CAD build for the part. Positions are in the model's coordinates, mm. Face numbers are marked on the shaded views. Give positions to 0.01 mm unless a question says otherwise; leave off trailing zeros. Order: outer loops, then holes, each group sorted by start corner. A loop starts at its lowest first (then second) coordinate and runs counter-clockwise, first axis right, second up.
Item 1: Two-plate mould, pull along X, no slides. Class the marked faces 1, 2 and 3: released by +X, released by -X, zero draft, split by the parting line, or undercut.
Item 2: Wall check: L1, parallel to Y at x = -1.8, z = 5.5; L2, parallel to Y at x = 1.3, z = -3.8; L3, parallel to Z at x = -0.25, y = 6. Give the ranges that are in metal, low to high.
Item 3: Band-saw the part on B-B on z = 7.75. Give the cut face in (x, y).
Item 4: Band-saw the part on C-C on y = 0. Give the cut face in (x, z), plus the area to 3 significant figures.
Item 5: Flat gauge pins, fed straight in: P1, Ø6.5, axis at x = -2.5, y = 3, coming from the -Z side; P2, Ø6, axis at y = -3, z = 2, coming from the +X side; P3, Ø0.6, axis at y = 0, z = -1.5, coming from the +X side. Where does each tip first touch, or does it go through?
Item 6: Band-saw the part on A-A on z = -3.8. Give the cut face in (x, y), plus the area to 3 significant figures.
```python
from build123d import *

# Parameters (mm, degrees)
ESQUISSE1_R             = 7
BOSS_EXTRU_1_DEPTH      = 12.5
ESQUISSE2_R             = 7
ESQUISSE2_R_2           = 6.4
ENL_V_MAT_EXTRU_1_DEPTH = 10.5
ESQUISSE4_R             = 3.15
ENL_V_MAT_EXTRU_3_DEPTH = 9
ESQUISSE5_R             = 0.8
BOSS_EXTRU_2_DEPTH      = 8.5
ESQUISSE6_W             = 0.5
ESQUISSE6_H             = 2
BOSS_EXTRU_3_DEPTH      = 5
ESQUISSE7_R             = 0.5
ENL_V_MAT_EXTRU_4_DEPTH = 9.587227572
ESQUISSE8_R             = 0.5
ENL_V_MAT_EXTRU_5_DEPTH = 12.087439586
CONG_7_R                = 0.8


with BuildPart() as part:
    # Esquisse1 → Boss.-Extru.1 (new body)
    with BuildSketch(Plane.XY):
        Circle(ESQUISSE1_R)
    extrude(amount=BOSS_EXTRU_1_DEPTH)

    # Esquisse2 → Enlèv. mat.-Extru.1 (cut)
    with BuildSketch(Plane(origin=(0, 0, 0), x_dir=(-1, 0, 0), z_dir=(0, 0, -1))):
        Circle(ESQUISSE2_R)
        Circle(ESQUISSE2_R_2, mode=Mode.SUBTRACT)
    extrude(amount=-ENL_V_MAT_EXTRU_1_DEPTH, mode=Mode.SUBTRACT)

    # Esquisse4 → Enlèv. mat.-Extru.3 (cut)
    with BuildSketch(Plane.XY.offset(12.5)):
        with Locations((-1.8, 0)):
            Circle(ESQUISSE4_R)
    extrude(amount=-ENL_V_MAT_EXTRU_3_DEPTH, mode=Mode.SUBTRACT)

    # Esquisse5 → Boss.-Extru.2 (add)
    with BuildSketch(Plane.XY.offset(3.5)):
        with Locations((-1.8, 0)):
            Circle(ESQUISSE5_R)
    extrude(amount=BOSS_EXTRU_2_DEPTH)

    # Esquisse6 → Boss.-Extru.3 (add)
    with BuildSketch(Plane(origin=(0, 0, 0), x_dir=(-1, 0, 0), z_dir=(0, 0, -1))):
        with Locations((-3.837439586, 0)):
            Rectangle(ESQUISSE6_W, ESQUISSE6_H)
        with Locations((-1.337227572, -3.389935619)):
            Rectangle(ESQUISSE6_W, ESQUISSE6_H)
    extrude(amount=BOSS_EXTRU_3_DEPTH)

    # Esquisse7 → Enlèv. mat.-Extru.4 (cut, through all)
    with BuildSketch(Plane(origin=(1.587227572, 0, 0), x_dir=(0, 0, -1), z_dir=(1, 0, 0))):
        with Locations((3.8, -3.389935619)):
            Circle(ESQUISSE7_R)
    extrude(amount=-ENL_V_MAT_EXTRU_4_DEPTH, mode=Mode.SUBTRACT)

    # Esquisse8 → Enlèv. mat.-Extru.5 (cut, through all)
    with BuildSketch(Plane(origin=(4.087439586, 0, 0), x_dir=(0, 0, -1), z_dir=(1, 0, 0))):
        with Locations((3.8, 0)):
            Circle(ESQUISSE8_R)
    extrude(amount=-ENL_V_MAT_EXTRU_5_DEPTH, mode=Mode.SUBTRACT)

    # Congé7
    cong_7_edges = [part.edges().sort_by_distance(p)[0] for p in [
        (-7, 0, 12.5),
    ]]
    fillet(cong_7_edges, radius=CONG_7_R)


solid = part.part
```
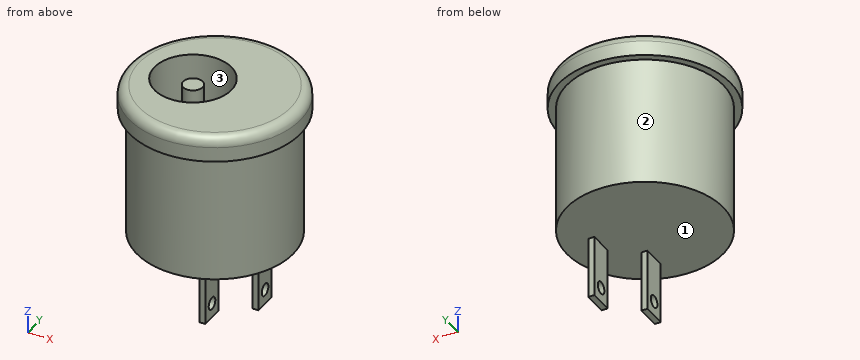
The answers:
1. face 1: zero draft
1. face 2: split by the parting line
1. face 3: undercut
2. L1: y = -6.14 to -3.15, -0.8 to 0.8, 3.15 to 6.14
2. L2: y = -4.39 to -3.89, -2.89 to -2.39
2. L3: z = 0 to 12.5
3. outline: circle Ø12.8 at (0, 0); circle Ø1.6 at (-1.8, 0); hole circle Ø6.3 at (-1.8, 0)
4. outline: (-7, 10.5) - (-6.4, 10.5) - (-6.4, 0) - (3.59, 0) - (3.59, -3.3) - (4.09, -3.3) - (4.09, 0) - (6.4, 0) - (6.4, 10.5) - (7, 10.5) - (7, 11.7) arc R0.8 ccw to (6.2, 12.5) - (1.35, 12.5) - (1.35, 3.5) - (-1, 3.5) - (-1, 12) - (-2.6, 12) - (-2.6, 3.5) - (-4.95, 3.5) - (-4.95, 12.5) - (-6.2, 12.5) arc R0.8 ccw to (-7, 11.7) - close; (3.59, -5) - (4.09, -5) - (4.09, -4.3) - (3.59, -4.3) - close
4. area: 121 mm2
5. P1: stops at z = 0
5. P2: stops at x = 6.4
5. P3: stops at x = 4.09
6. outline: (1.09, -4.39) - (1.59, -4.39) - (1.59, -3.89) - (1.09, -3.89) - close; (1.09, -2.89) - (1.59, -2.89) - (1.59, -2.39) - (1.09, -2.39) - close; (3.59, -1) - (4.09, -1) - (4.09, -0.5) - (3.59, -0.5) - close; (3.59, 0.5) - (4.09, 0.5) - (4.09, 1) - (3.59, 1) - close
6. area: 1.00 mm2
